Check sheet for the drawn part. Datum: minimum x, y, z corner. Units: mm. A direction names the side the tool comes from. Give positions to 0.01 mm unless a question says otherwise; leave off trailing zeros. Write each loop counter-clockwise with the first axis right and the second up, starting at its lowest first coordinate (ties: lowest second). Pieces come first, ordered by that corner, then holes.
(1) Cross-section at C-C (z = 49). Record the boundary of the cut face in (x, y), and give its area (3 significant figures).
(2) Cross-section at B-B (x = 154.5). Record the boundary of the cut face in (y, z) (3 decimals).
(3) Depth check by flat-ended pin: P1, Ø21, axis at y = 32, z = 52, coming from the -X side; P2, Ø12.5, axis at x = 247, y = 19, coming from the -Z side; P3, Ø5.5, axis at y = 30.5, z = 54.5, coming from the +X side; P4, Ø12.5, axis at x = 253, y = 65.5, coming from the -Z side. Enter the tip coordinate at first touch or a pass-through.
(4) Thickness scan on line 1 along Z through (x, y) = (381, 20) (3 decimals); line 2 along Z through (x, y) = (283.5, 73) (3 decimals); line 3 along X through (y, z) = (77, 44). Record the ranges inside material, lowest first.
(5) Tool access check on the marked faces 1, 2 and 3. Record the directions out of +Z, -Z, +X, -X, +Y, -Y that give a thin tool (end or side, any length) a straight path to the whole face; none if there is none.
(6) Cross-section at A-A (y = 80). Record the boundary of the cut face in (x, z) (3 decimals).
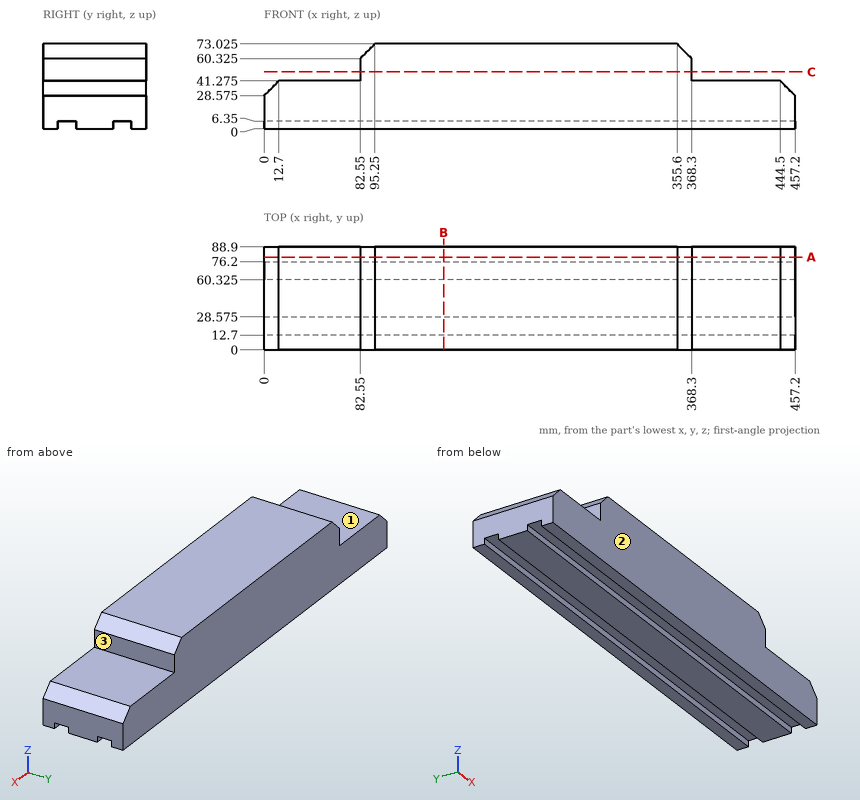
Reply:
1. outline: (82.55, 0) - (368.3, 0) - (368.3, 88.9) - (82.55, 88.9) - close
1. area: 25,400 mm2
2. outline: (0, 0) - (12.7, 0) - (12.7, 6.35) - (28.575, 6.35) - (28.575, 0) - (60.325, 0) - (60.325, 6.35) - (76.2, 6.35) - (76.2, 0) - (88.9, 0) - (88.9, 73.025) - (0, 73.025) - close
3. P1: stops at x = 82.55
3. P2: stops at z = 6.35
3. P3: stops at x = 368.3
3. P4: stops at z = 0
4. line 1: z = 6.35 to 41.275
4. line 2: z = 6.35 to 73.025
4. line 3: x = 82.55 to 368.3
5. face 1: +Z, -X, +Y, -Y
5. face 2: +Z, -Z, +X, -X, -Y
5. face 3: +Z, +X, +Y, -Y
6. outline: (0, 0) - (457.2, 0) - (457.2, 28.575) - (444.5, 41.275) - (368.3, 41.275) - (368.3, 60.325) - (355.6, 73.025) - (95.25, 73.025) - (82.55, 60.325) - (82.55, 41.275) - (12.7, 41.275) - (0, 28.575) - close
